```python
from build123d import *

# Parameters (mm, degrees)
SKETCH1_R           = 3.2639
SKETCH1_R_2         = 2.0193
SKETCH1_R_3         = 215.9
BOSS_EXTRUDE1_DEPTH = 3.175


with BuildPart() as part:
    # Sketch1 → Boss-Extrude1 (new body)
    with BuildSketch(Plane(origin=(0, 0, 0), x_dir=(1, 0, 0), z_dir=(0, 1, 0))):
        with BuildLine():
            ThreePointArc((241.3, 0), (39.144028917, 238.103832393), (-228.600000001, 77.251084131))
            Line((-228.6, 77.251084131), (-228.6, -77.251084131))
            ThreePointArc((-228.600000001, -77.251084131), (39.144028917, -238.103832393), (241.3, 0))
        make_face()
        with Locations((0, -228.6)):
            Circle(SKETCH1_R, mode=Mode.SUBTRACT)
        with Locations((-197.973407305, -114.3)):
            Circle(SKETCH1_R, mode=Mode.SUBTRACT)
        with Locations((-215.9, -63.5)):
            Circle(SKETCH1_R_2, mode=Mode.SUBTRACT)
        with Locations((197.973407305, -114.3)):
            Circle(SKETCH1_R, mode=Mode.SUBTRACT)
        with Locations((228.6, -12.7)):
            Circle(SKETCH1_R_2, mode=Mode.SUBTRACT)
        with Locations((-215.9, 63.5)):
            Circle(SKETCH1_R_2, mode=Mode.SUBTRACT)
        with Locations((-197.973407305, 114.3)):
            Circle(SKETCH1_R, mode=Mode.SUBTRACT)
        Circle(SKETCH1_R_3, mode=Mode.SUBTRACT)
        with Locations((0, 228.6)):
            Circle(SKETCH1_R, mode=Mode.SUBTRACT)
        with Locations((197.973407305, 114.3)):
            Circle(SKETCH1_R, mode=Mode.SUBTRACT)
        with Locations((228.6, 0)):
            Circle(SKETCH1_R_2, mode=Mode.SUBTRACT)
        with Locations((228.6, 12.7)):
            Circle(SKETCH1_R_2, mode=Mode.SUBTRACT)
    extrude(amount=BOSS_EXTRUDE1_DEPTH)


solid = part.part
```
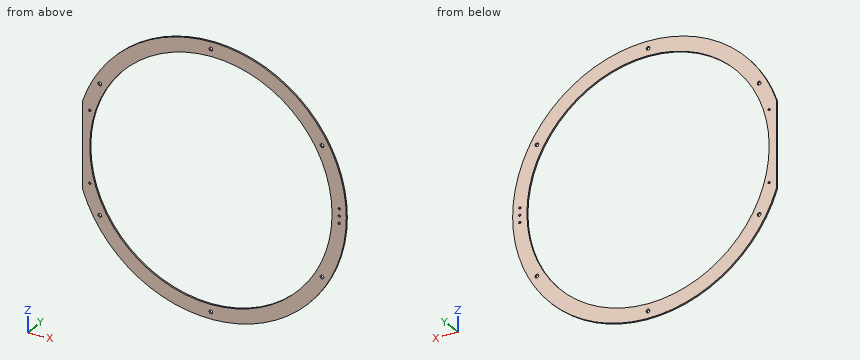
Verification items for the finished model (mm, model axes). Round coordinates to 2 decimals unless told otherwise and drop trailing zeros. Write each loop counter-clockwise with the first axis right and the second up, starting at its lowest first coordinate (ties: lowest second). Pieces come first, ordered by that corner, then holes. Notation, with made-up numbers: (63.5, -15.5) - (94.5, -15.5) arc R7 cw to (94.5, -11.5) - close; hole circle Ø9 at (77.25, 62). An arc over 180 degrees is marked (long way). Answer as a JSON object with one key per item and string values. Group by question number.
Q1. Section check C-C, the plane x = 168.5. Enter the section's corners in (y, z) (3 decimals).
Q2. Section check A-A, the plane y = 2.65. Give the number of separate pieces and of enclosed holes in the cut face, plus the area to 3 significant figures.
Q3. Section check B-B, the plane z = 152. Enter the section's corners in (x, y) (3 decimals), plus the area to 3 significant figures.
Q4. Go/stop test with flat-tipped pins: pin 1 Ø6 at (x, z) = (-197.97, 114.3) entering from +Y; pin 2 Ø1.5 at (x, y) = (-61.5, 1.5) entering from +Z. Record where each tip stops, or that it passes through.
Q5. Thickness scan on line 1 (Z direction, x = 0, y = 0.75); line 2 (X direction, y = 2, z = -12.7); line 3 (Z direction, x = 198.5, y = 0.35). Record the ranges inside material, lowest first.
Found:
{
 "1": {"outline": "(0, -172.724) - (3.175, -172.724) - (3.175, -134.984) - (0, -134.984) - close; (0, 134.984) - (3.175, 134.984) - (3.175, 172.724) - (0, 172.724) - close"},
 "2": {"separate pieces": "1", "enclosed holes": "12", "area": "34,900 mm^2"},
 "3": {"outline": "(-187.408, 0) - (-153.326, 0) - (-153.326, 3.175) - (-187.408, 3.175) - close; (153.326, 0) - (187.408, 0) - (187.408, 3.175) - (153.326, 3.175) - close", "area": "216 mm^2"},
 "4": {"pin 1": "passes through", "pin 2": "stops at z = 233.53"},
 "5": {"line 1": "z = -241.3 to -231.86, -225.34 to -215.9, 215.9 to 225.34, 231.86 to 241.3", "line 2": "x = -228.6 to -215.53, 215.53 to 226.58, 230.62 to 240.97", "line 3": "z = -137.2 to -117.52, -111.08 to -84.92, 84.92 to 111.08, 117.52 to 137.2"}
}
